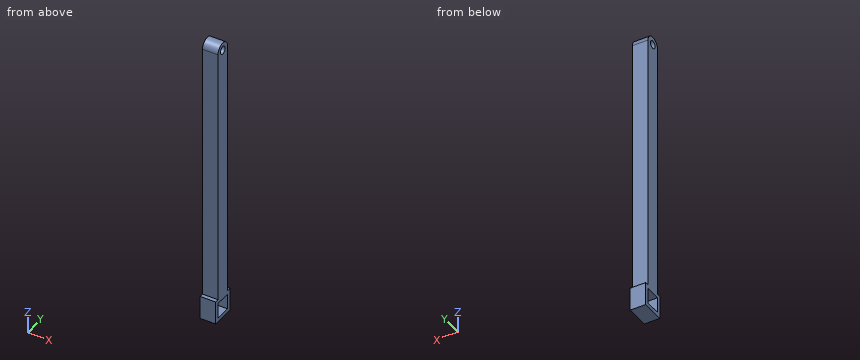
Autodesk Inventor part; units mm, degrees
ref_plane "YZ Plane" through (0, 0, 0) normal (1, 0, 0) x (0, 1, 0)
ref_plane "XZ Plane" through (0, 0, 0) normal (0, 1, 0) x (-1, 0, 0)
ref_plane "XY Plane" through (0, 0, 0) normal (0, 0, 1) x (1, 0, 0)
sketch "Sketch1" plane through (0, 0, 0) normal (1, 0, 0) x (0, 1, 0)
  arc A0 (0, 266.1728) -> (-40, 266.1728) centre (-20, 266.1728) ccw
  circle A1 centre (-20, 266.1728) radius 10
  line L0 (0, 266.1728) -> (-10, 266.1728)
  line L1 (-0.0023, -412.6691) -> (-40.0023, -412.6691)
  line L2 (-40.0023, -412.6691) -> (-40.0023, -452.6691)
  line L3 (-40.0023, -452.6691) -> (-0.0023, -452.6691)
  line L4 (-0.0023, -452.6691) -> (-0.0023, -412.6691)
  line L5 (-50, -462.6691) -> (10, -462.6691)
  line L6 (10, -462.6691) -> (10, -402.6691)
  line L7 (10, -402.6691) -> (-50, -402.6691)
  line L8 (-50, -402.6691) -> (-50, -462.6691)
  line L9 (-40, 266.1728) -> (-40, -402.6691)
  line L10 (0, -402.6691) -> (0, 266.1728)
  point P0 (0, 0)
  dimension "d5" = 20
  dimension "d4" = 40
  dimension "d6" = 40
  dimension "d7" = 40
  dimension "d8" = 60
  dimension "d9" = 60
  dimension "d11" = 10
  dimension "d13" = 20
extrude "Extrusion1" add sketch "Sketch1" along normal blind 40
properties part number "long extention"
Here's how the part is built. I have some questions about the finished solid (model axes, mm). Round coordinates to 2 decimals unless told otherwise and drop trailing zeros. Loops run counter-clockwise (first coordinate to the right, second up) from the corner with the lowest first, then second, coordinate; pieces in that order, holes last. Notation, with made-up numbers: (7.25, 33.5) - (38.25, 33.5) arc R21 ccw to (38.25, 63.5) - close; hole circle Ø8 at (-39, 56). An arc over 180 degrees is marked (long way). One line per question, with ' | ' between items. Start each with the question number.
Q1. I want a section at B-B (x = 9.5). Write out the boundary of the cut face in (y, z), then the cut area to 3 significant figures.
Q2. I want a section at A-A (y = -20). Write out the boundary of the cut face in (x, z), then the cut area to 3 significant figures.
Q3. Will these pins go through, and if not, where does the flat tip stop? pin 1 (12 mm diameter, centred on x = 5.5, y = -9, fed in from +Z); pin 2 (10 mm diameter, centred on x = 24, z = -86.5, fed in from +Y); pin 3 (5 mm diameter, centred on x = 30, y = 4.5, fed in from +Z).
Q4. I want a section at C-C (z = -294.5). Write out the boundary of the cut face in (x, y), then the cut area to 3 significant figures.
Q5. Please list where these lines run through material, in increasing order: line 1 (Z direction, x = 9, y = -20); line 2 (Z direction, x = 18.5, y = -22.5); line 3 (Y direction, x = 9, z = -200). Write a range as [from, to].
Response values:
1) outline: (-50, -462.67) - (10, -462.67) - (10, -402.67) - (0, -402.67) - (0, 266.17) arc R20 ccw to (-40, 266.17) - (-40, -402.67) - (-50, -402.67) - close; hole (-40, -452.67) - (0, -452.67) - (0, -412.67) - (-40, -412.67) - close; hole circle Ø20 at (-20, 266.17) | area: 29,100 mm²
2) outline: (0, -462.67) - (40, -462.67) - (40, -452.67) - (0, -452.67) - close; (0, -412.67) - (40, -412.67) - (40, 256.17) - (0, 256.17) - close; (0, 276.17) - (40, 276.17) - (40, 286.17) - (0, 286.17) - close | area: 27,600 mm²
3) pin 1: stops at z = 285.54 | pin 2: stops at y = 0 | pin 3: stops at z = -402.67
4) outline: (0, -40) - (40, -40) - (40, 0) - (0, 0) - close | area: 1,600 mm²
5) line 1: z = [-462.67, -452.67], [-412.67, 256.17], [276.17, 286.17] | line 2: z = [-462.67, -452.67], [-412.67, 256.49], [275.86, 286.02] | line 3: y = [-40, 0]
